```python
from build123d import *

# Parameters (mm, degrees)
F0_W     = 95
F0_H     = 54
F1_DEPTH = 8.5
F3_DEPTH = 7
F4_W     = 2
F4_H     = 18.1
F5_DEPTH = 7
F7_DEPTH = 5


with BuildPart() as f1:
    # F0 (on Top) → F1 (new body)
    with BuildSketch(Plane.XY):
        Rectangle(F0_W, F0_H)
    extrude(amount=F1_DEPTH)

    # F2 (on face) → F3 (cut)
    with BuildSketch(Plane.XY.offset(8.5)):
        Polygon((-45.5, 25), (-45.5, -25), (45.5, -25), (45.5, 25), (36.37, 25), (36.37, 16.354831), (35.37, 16.354831), (35.37, 25), (25.32, 25), (25.32, 16.354831), (24.32, 16.354831), (24.32, 25), (16.26, 25), (16.26, 16.354831), (15.26, 16.354831), (15.26, 25), (5.62, 25), (5.62, 16.354831), (4.62, 16.354831), (4.62, 25), align=None)
    extrude(amount=-F3_DEPTH, mode=Mode.SUBTRACT)

    # F4 (on face) → F5 (cut)
    with BuildSketch(Plane.XY.offset(8.5)):
        with Locations((-46.5, -3.35)):
            Rectangle(F4_W, F4_H)
    extrude(amount=-F5_DEPTH, mode=Mode.SUBTRACT)

    # F6 (on face) → F7 (cut)
    with BuildSketch(Plane.XY.offset(8.5)):
        Polygon((46.5, -26), (-46.5, -26), (-46.5, -12.4), (-47.5, -12.4), (-47.5, -27), (47.5, -27), (47.5, 27), (-47.5, 27), (-47.5, 5.7), (-46.5, 5.7), (-46.5, 26), (46.5, 26), align=None)
    extrude(amount=-F7_DEPTH, mode=Mode.SUBTRACT)


solid = f1.part
```
For this review, take the finished solid that the model builds, in its own axes (mm). A direction names the side the tool comes from. Coordinates: 2 decimals unless noted, no trailing zeros. Order: outer loops, then holes, each group sorted by start corner. A loop starts at its lowest first (then second) coordinate and runs counter-clockwise, first axis right, second up. Notation, with made-up numbers: (42, 18.5) -> (57, 18.5) arc R24 cw to (57, 49.5) -> close; hole circle Ø2 at (32, 28.25). An arc over 180 degrees is marked (long way). Use CSV: the item, a comma, the result in double quotes. Start each with the question number.
Item 1: We need section B-B, the plane y = 20.5. Give the boundary of the cut face in (x, z), then the cut area to 4 significant figures.
Item 2: Wall thickness on probe 1 along X at (y, z) = (17, 7); probe 2 along X at (y, z) = (14, 8.25); probe 3 along Y at (x, z) = (-29, 2.5): over which ranges is each line inside the solid? List them lowest first.
Item 3: We need section C-C, the plane x = -32. Give the boundary of the cut face in (y, z), then the cut area to 3 significant figures.
Item 4: We need section A-A, the plane z = 5. Give the boundary of the cut face in (x, y).
Item 5: Draft analysis for pull direction Y (two halves, no side actions). For faces 1 (the face through (25.32, 21, 5)), 2 (the face through (-46.5, -19, 6)), 3 (the face through (-1, 27, 2)), state which applies: pulls with the +Y half, pulls with the -Y half, needs draft (parallel to the pull), parting line crosses it, or undercut.
Item 6: We need section D-D, the plane y = -14. Give the boundary of the cut face in (x, z).
Item 7: For faces 4 (the face through (5.62, 21, 5)), 5 (the face through (-46.5, 16, 6)), 6 (the face through (-1, 26, 6)), list the 3-axis set-ups (+Z, -Z, +X, -X, +Y, -Y) from which the entire face can be reached by the end or side of a thin tool; tool diameter is ignored.
Item 8: Insertion check: pin 1 (3 mm diameter, centred on y = -9, z = 2.5, fed in from -X); pin 2 (1.5 mm diameter, centred on y = -18, z = 5.5, fed in from -X); pin 3 (3 mm diameter, centred on y = -21, z = 7, fed in from +X); pin 4 (15 mm diameter, centred on x = -16, y = -10, fed in from +Z). Each pin has a flat end and moves straight along its axis. Give the tip position at first contact, or say it passes through.
Derived:
1,outline,"(-47.5, 0) -> (47.5, 0) -> (47.5, 3.5) -> (46.5, 3.5) -> (46.5, 8.5) -> (45.5, 8.5) -> (45.5, 1.5) -> (36.37, 1.5) -> (36.37, 8.5) -> (35.37, 8.5) -> (35.37, 1.5) -> (25.32, 1.5) -> (25.32, 8.5) -> (24.32, 8.5) -> (24.32, 1.5) -> (16.26, 1.5) -> (16.26, 8.5) -> (15.26, 8.5) -> (15.26, 1.5) -> (5.62, 1.5) -> (5.62, 8.5) -> (4.62, 8.5) -> (4.62, 1.5) -> (-45.5, 1.5) -> (-45.5, 8.5) -> (-46.5, 8.5) -> (-46.5, 3.5) -> (-47.5, 3.5) -> close"
1,area,"188.5 mm^2"
2,probe 1,"x = -46.5 to -45.5, 4.62 to 5.62, 15.26 to 16.26, 24.32 to 25.32, 35.37 to 36.37, 45.5 to 46.5"
2,probe 2,"x = -46.5 to -45.5, 45.5 to 46.5"
2,probe 3,"y = -27 to -25, 25 to 27"
3,outline,"(-27, 0) -> (27, 0) -> (27, 3.5) -> (26, 3.5) -> (26, 8.5) -> (25, 8.5) -> (25, 1.5) -> (-25, 1.5) -> (-25, 8.5) -> (-26, 8.5) -> (-26, 3.5) -> (-27, 3.5) -> close"
3,area,"99.0 mm^2"
4,outline,"(-46.5, -26) -> (46.5, -26) -> (46.5, 26) -> (-46.5, 26) -> (-46.5, 5.7) -> (-45.5, 5.7) -> (-45.5, 25) -> (4.62, 25) -> (4.62, 16.35) -> (5.62, 16.35) -> (5.62, 25) -> (15.26, 25) -> (15.26, 16.35) -> (16.26, 16.35) -> (16.26, 25) -> (24.32, 25) -> (24.32, 16.35) -> (25.32, 16.35) -> (25.32, 25) -> (35.37, 25) -> (35.37, 16.35) -> (36.37, 16.35) -> (36.37, 25) -> (45.5, 25) -> (45.5, -25) -> (-45.5, -25) -> (-45.5, -12.4) -> (-46.5, -12.4) -> close"
5,face 1,"undercut"
5,face 2,"needs draft"
5,face 3,"pulls with the +Y half"
6,outline,"(-47.5, 0) -> (47.5, 0) -> (47.5, 3.5) -> (46.5, 3.5) -> (46.5, 8.5) -> (45.5, 8.5) -> (45.5, 1.5) -> (-45.5, 1.5) -> (-45.5, 8.5) -> (-46.5, 8.5) -> (-46.5, 3.5) -> (-47.5, 3.5) -> close"
7,face 4,"+Z"
7,face 5,"+Z, -X, +Y, -Y"
7,face 6,"+Z, +X, -X, +Y"
8,pin 1,"stops at x = -47.5"
8,pin 2,"stops at x = -46.5"
8,pin 3,"stops at x = 46.5"
8,pin 4,"stops at z = 1.5"
